Autodesk Inventor part; units mm, degrees
ref_plane "YZ Plane" through (0, 0, 0) normal (1, 0, 0) x (0, 1, 0)
ref_plane "XZ Plane" through (0, 0, 0) normal (0, 1, 0) x (-1, 0, 0)
ref_plane "XY Plane" through (0, 0, 0) normal (0, 0, 1) x (1, 0, 0)
sketch "Sketch1" plane through (0, 0, 0) normal (0, 1, 0) x (-1, 0, 0)
  circle A0 centre (0, 0) radius 50.8
  dimension "d0" = 101.6
extrude "Extrusion1" add sketch "Sketch1" along normal blind 5.588
sketch "Sketch2" plane through (0, 5.588, 0) normal (0, 1, 0) x (1, 0, 0)
  circle A0 centre (0, 17.78) radius 0.635
  point P0 (0, 0)
  dimension "d3" = 1.27
extrude "Extrusion2" cut sketch "Sketch2" against normal blind 5.588
sketch "Sketch3" plane through (0, 5.588, 0) normal (0, 1, 0) x (1, 0, 0)
  point P0 (0, 0)
sketch "Sketch4" plane through (0, 5.588, 0) normal (0, 1, 0) x (1, 0, 0)
  circle A0 centre (0, -17.78) radius 0.635
  point P0 (0, 0)
  dimension "d6" = 1.27
extrude "Extrusion3" cut sketch "Sketch4" against normal blind 5.588
properties part number "outerCup"
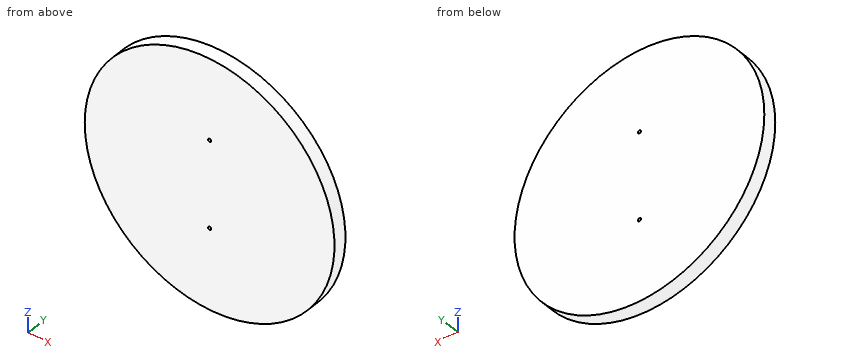
The model under review builds one solid part; all positions refer to its coordinate system, in mm. Give positions to 0.01 mm unless a question says otherwise; leave off trailing zeros. Order: outer loops, then holes, each group sorted by start corner. A loop starts at its lowest first (then second) coordinate and runs counter-clockwise, first axis right, second up. Notation, with made-up numbers: (-14.75, 62.5) - (-7.75, 62.5) arc R7 cw to (-7.75, 74.5) - close; hole circle Ø5 at (78.25, 60.25). An arc over 180 degrees is marked (long way). Use CSV: the item, a comma, the result in double quotes. Start each with the question number.
Q1. We need section B-B, the plane x = -34. Write out the cut boundary in (y, z), and give its area (3 significant figures).
Q2. To check wall thickness, follow line 1 along Z through (x, y) = (0, 2.35) (3 decimals); line 2 along X through (y, z) = (4, -17.78) (3 decimals); line 3 along X through (y, z) = (2.15, -9). State the ranges of each line that lie inside material, in increasing order. Write a range as [from, to].
Q3. Clearance check with flat-ended pins moving along their axes: pin 1 Ø12 at (x, z) = (-34.5, -26.5) entering from -Y; pin 2 Ø0.8 at (x, z) = (0, 17.78) entering from +Y; pin 3 Ø1.5 at (y, z) = (1.5, -22) entering from +X. State where each tip first meets the part, or that it passes through.
Q4. We need section C-C, the plane z = 12. Write out the cut boundary in (x, y), and give its area (3 significant figures).
Q5. We need section A-A, the plane y = 3.2. Write out the cut boundary in (x, z) (3 decimals).
Outcome:
1,outline,"(0, -37.74) - (5.59, -37.74) - (5.59, 37.74) - (0, 37.74) - close"
1,area,"422 mm^2"
2,line 1,"z = [-50.8, -18.415], [-17.145, 17.145], [18.415, 50.8]"
2,line 2,"x = [-47.587, -0.635], [0.635, 47.587]"
2,line 3,"x = [-50, 50]"
3,pin 1,"stops at y = 0"
3,pin 2,"passes through"
3,pin 3,"stops at x = 46.14"
4,outline,"(-49.36, 0) - (49.36, 0) - (49.36, 5.59) - (-49.36, 5.59) - close"
4,area,"552 mm^2"
5,outline,"circle Ø101.6 at (0, 0); hole circle Ø1.27 at (0, -17.78); hole circle Ø1.27 at (0, 17.78)"
